Could you check a few things on this drawing? It's one solid part, dimensions in mm from its lowest x, y, z. A direction names the side the tool comes from. Round coordinates to 2 decimals unless told otherwise and drop trailing zeros. Order: outer loops, then holes, each group sorted by start corner. A loop starts at its lowest first (then second) coordinate and runs counter-clockwise, first axis right, second up. Notation, with made-up numbers: (58.5, -1.75) - (69.5, -1.75) arc R23 cw to (69.5, 33.25) - close; hole circle Ø11 at (4, 16). An arc over 180 degrees is marked (long way). Use one line per item in the form item = value.
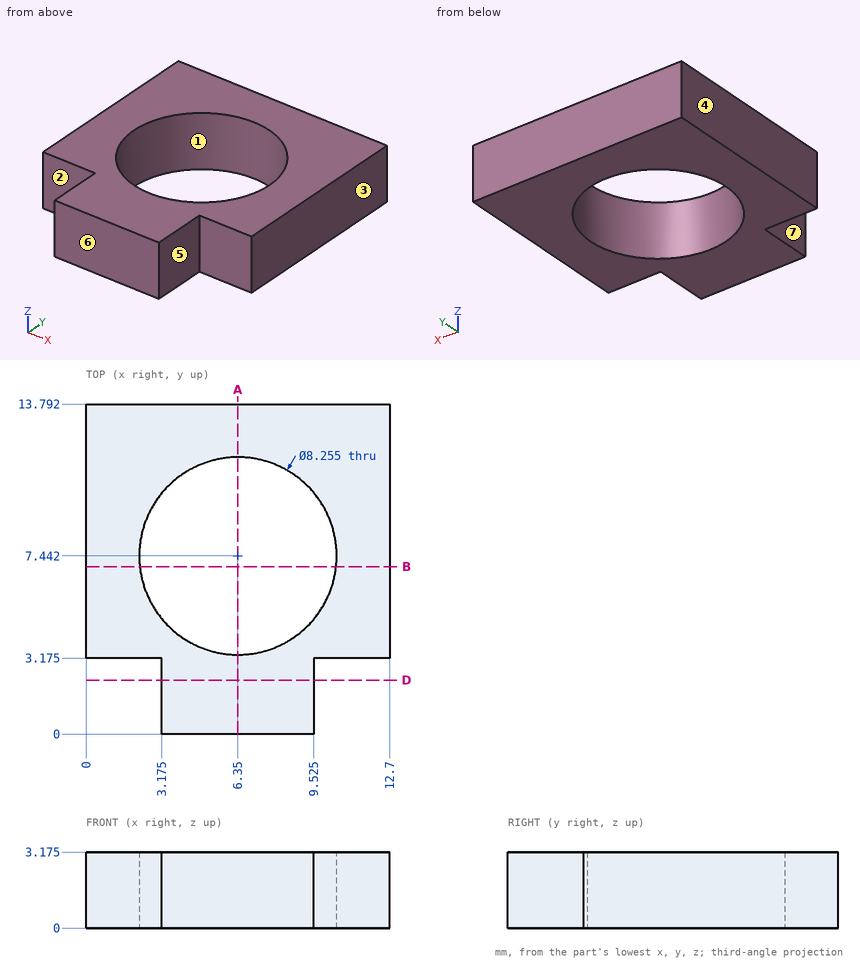
Item 1: I need wall thicknesses on L1, parallel to Y at x = 6.35, z = 2.35 (1 decimal); L2, parallel to X at y = 6.75, z = 0.25; L3, parallel to X at y = 1, z = 0.85 (3 decimals). Which ranges of each line are inside material? Lowest first, please.
Found:
L1 = 0 to 3.3, 11.6 to 13.8
L2 = 0 to 2.28, 10.42 to 12.7
L3 = 3.175 to 9.525
Item 2: If we mould it in two halves opening along X, with no side actions, what happens to the marked faces 1, 2, 3 and 4? For each: released by +X, released by -X, zero draft, split by the parting line, or undercut.
Found:
face_1 = undercut
face_2 = zero draft
face_3 = released by +X
face_4 = released by -X
Item 3: Imagine slicing it at D-D on y = 2.25. Please give me the cut outline in (x, z) (3 decimals), plus the area to 3 significant figures.
Found:
outline = (3.175, 0) - (9.525, 0) - (9.525, 3.175) - (3.175, 3.175) - close
area = 20.2 mm2
Item 4: Imagine slicing it at A-A on x = 6.35. Please give me the cut outline in (y, z) (1 decimal), plus the area to 3 significant figures.
Found:
outline = (0, 0) - (3.3, 0) - (3.3, 3.2) - (0, 3.2) - close; (11.6, 0) - (13.8, 0) - (13.8, 3.2) - (11.6, 3.2) - close
area = 17.6 mm2
Item 5: Will these pins go through, and if not, where does the flat tip stop? P1, Ø1, axis at x = 1.5, z = 2, coming from the -Y side (3 decimals); P2, Ø1.6, axis at y = 2, z = 1, coming from the +X side (3 decimals).
Found:
P1 = 3.175
P2 = 9.525
Item 6: Imagine slicing it at B-B on y = 7. Please give me the cut outline in (x, z) (1 decimal), plus the area to 3 significant figures.
Found:
outline = (0, 0) - (2.2, 0) - (2.2, 3.2) - (0, 3.2) - close; (10.5, 0) - (12.7, 0) - (12.7, 3.2) - (10.5, 3.2) - close
area = 14.3 mm2
Item 7: For the marked faces 5, 6 and 7, which set-ups out of +Z, -Z, +X, -X, +Y, -Y let a thin tool reach every point of the face, with its end or its side?
Found:
face_5 = +Z, -Z, +X, -Y
face_6 = +Z, -Z, +X, -X, -Y
face_7 = +Z, -Z, -X, -Y
